Geometry check sheet. Reference: the model listing, model coordinates, mm. Coordinates: 2 decimals unless noted, no trailing zeros. Write each loop counter-clockwise with the first axis right and the second up, starting at its lowest first coordinate (ties: lowest second). Pieces come first, ordered by that corner, then holes.
from build123d import *

# Parameters (mm, degrees)
F3_DEPTH  = 27
F3_FACE_W = 0.5
F3_FACE_H = 0.5
F4_DEPTH  = 1.5


with BuildPart() as f1:
    # F0 (on Front) → F1 (revolve)
    with BuildSketch(Plane.XZ):
        with BuildLine():
            Line((2.15, 1.45), (0, 1.45))
            ThreePointArc((0, 1.45), (-1.025305, 1.025305), (-1.45, 0))
            Line((-1.45, 0), (3.15, 0))
            Line((3.15, 0), (3.15, 1.6))
            Line((3.15, 1.6), (2.15, 1.6))
            Line((2.15, 1.6), (2.15, 1.45))
        make_face()
    revolve(axis=Axis((4.33001, 0, 0), (1, 0, 0)))

    # F2 (on face) → F3 (join)
    with BuildSketch(Plane.YZ.offset(3.15)):
        Polygon((0.25, -0.77), (-0.25, -0.77), (-0.25, -1.27), (0, -1.27), (0.25, -1.27), align=None)
        Polygon((0.25, 1.27), (0, 1.27), (-0.25, 1.27), (-0.25, 0.77), (0.25, 0.77), align=None)
    extrude(amount=F3_DEPTH)

    # F3_face (on face) → F4 (cut)
    with BuildSketch(Plane(origin=(30.15, 0, 1.02), x_dir=(0, 1, 0), z_dir=(1, 0, 0))):
        Rectangle(F3_FACE_W, F3_FACE_H)
    extrude(amount=-F4_DEPTH, mode=Mode.SUBTRACT)


solid = f1.part
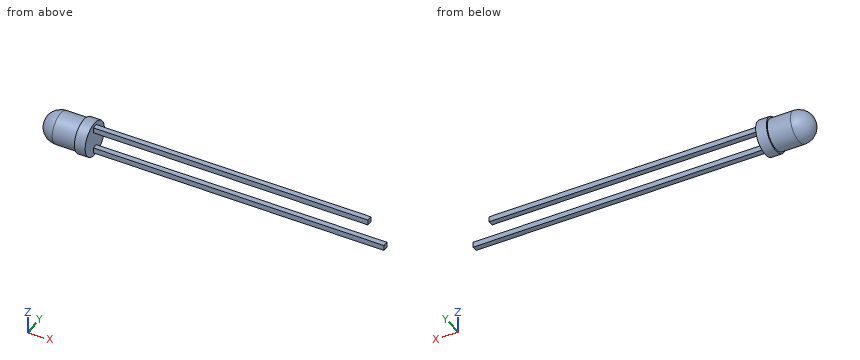
1. Sectioned sample at A-A, the plane x = 10. Record the boundary of the cut face in (y, z).
Computed values:
outline: (-0.25, -1.27) - (0.25, -1.27) - (0.25, -0.77) - (-0.25, -0.77) - close; (-0.25, 0.77) - (0.25, 0.77) - (0.25, 1.27) - (-0.25, 1.27) - close
2. Sectioned sample at B-B, the plane x = 0.5. Record the boundary of the cut face in (y, z), and give its area (3 significant figures).
Computed values:
outline: circle Ø2.9 at (0, 0)
area: 6.61 mm2
3. Thickness scan on line 1 along Z through (x, y) = (3.5, -0.2); line 2 along X through (y, z) = (0.1, 0.05); line 3 along Y through (x, z) = (25.5, 1.2). Record the ranges inside material, lowest first.
Computed values:
line 1: z = -1.27 to -0.77, 0.77 to 1.27
line 2: x = -1.45 to 3.15
line 3: y = -0.25 to 0.25
4. Gauge pin test, flat ends, axial feed: pin 1 Ø1.5 at (y, z) = (0, 1) entering from +X; pin 2 Ø1 at (y, z) = (0.5, 0.5) entering from -X; pin 3 Ø0.6 at (x, y) = (19, 0) entering from -Z. Record the tip position at first contact, or that the pin passes through.
Computed values:
pin 1: stops at x = 28.65
pin 2: stops at x = -1.44
pin 3: stops at z = -1.27
